```python
from build123d import *

# Parameters (mm, degrees)
F0_W     = 1701.8
F0_H     = 1422.4
F1_DEPTH = 1422.4
F3_DEPTH = 160.02
F4_W     = 736.6
F4_H     = 83.82
F5_DEPTH = 1701.8
F6_R     = 381
F7_DEPTH = 3035.3


with BuildPart() as f1:
    # F0 (on Front) → F1 (new body)
    with BuildSketch(Plane.XZ):
        Rectangle(F0_W, F0_H)
    extrude(amount=F1_DEPTH)

    # F2 (on face) → F3 (cut)
    with BuildSketch(Plane.XZ.offset(1422.4)):
        with BuildLine():
            ThreePointArc((63.5, 500.38), (44.901281, 545.281281), (0, 563.88))
            ThreePointArc((0, 563.88), (-44.901281, 455.478719), (63.5, 500.38))
        make_face()
    extrude(amount=-F3_DEPTH, mode=Mode.SUBTRACT)

    # F4 (on face) → F5 (cut)
    with BuildSketch(Plane.YZ.offset(850.9)):
        with Locations((-368.3, 351.79)):
            Rectangle(F4_W, F4_H)
    extrude(amount=-F5_DEPTH, mode=Mode.SUBTRACT)

    # F6 (on face) → F7 (cut)
    with BuildSketch(Plane.YZ.offset(850.9)):
        with Locations((-753.856719, -178.938612)):
            Circle(F6_R)
    extrude(amount=-F7_DEPTH, mode=Mode.SUBTRACT)


solid = f1.part
```
Geometry: final body of the model. Coordinates: model frame, mm. A direction names the side the tool comes from. Round coordinates to 2 decimals unless told otherwise and drop trailing zeros. Order: outer loops, then holes, each group sorted by start corner. A loop starts at its lowest first (then second) coordinate and runs counter-clockwise, first axis right, second up. Notation, with made-up numbers: (73, -9.5) -> (126, -9.5) arc R35 cw to (126, 27.5) -> close; hole circle Ø11 at (69, 50.25). An arc over 180 degrees is marked (long way). Use CSV: the item, a comma, the result in double quotes. Start each with the question number.
1) Section A-A (y = -140). Return the cut outline in (x, z).
2) First-contact query: pin 1 Ø25 at (x, z) = (151, 358.5) entering from +Y. Flat tip, straight axial feed; report the tip coordinate or a pass-through.
3) Set-up query: faces 4 (the face through (850.9, -543, 148)), 5 (the face through (12, -373, 393.7)). Return all of +Z, -Z, +X, -X, +Y, -Y with unobstructed straight access to the full face (end or side cutting, diameter ignored); none if empty.
4) Material intervals for line 1 along Y through (x, z) = (-549.5, -176); line 2 along X through (y, z) = (-1371.5, 500.38); line 3 along Y through (x, z) = (-560.5, 382), sorted ascending. Write a range as from..to.
5) Section B-B (z = 145.5). Return the cut outline in (x, y), and give its area (3 significant figures).
6) Section C-C (x = 583). Return the cut outline in (y, z).
7) Draft query along Z for faces 1 (the face through (-12, -701, -711.2)), 2 (the face through (-12, 0, -194)), 3 (the face through (-1, -1262.38, 501)). Return one class per face: +Z half, -Z half, draft (parallel to the pull), parting line (faces both ways), or undercut.
Returned:
1,outline,"(-850.9, -711.2) -> (850.9, -711.2) -> (850.9, 309.88) -> (-850.9, 309.88) -> close; (-850.9, 393.7) -> (850.9, 393.7) -> (850.9, 711.2) -> (-850.9, 711.2) -> close"
2,pin 1,"stops at y = -736.6"
3,face 4,"+Z, -Z, +X, +Y, -Y"
3,face 5,"+X, -X, +Y"
4,line 1,"y = -1422.4..-1134.85, -372.87..0"
4,line 2,"x = -850.9..-63.5, 63.5..850.9"
4,line 3,"y = -1422.4..-736.6"
5,outline,"(-850.9, -1422.4) -> (850.9, -1422.4) -> (850.9, -953.61) -> (-850.9, -953.61) -> close; (-850.9, -554.11) -> (850.9, -554.11) -> (850.9, 0) -> (-850.9, 0) -> close"
5,area,"1,740,000 mm²"
6,outline,"(-1422.4, -711.2) -> (0, -711.2) -> (0, 309.88) -> (-736.6, 309.88) -> (-736.6, 393.7) -> (0, 393.7) -> (0, 711.2) -> (-1422.4, 711.2) -> close; hole circle Ø762 at (-753.86, -178.94)"
7,face 1,"-Z half"
7,face 2,"draft"
7,face 3,"undercut"
